For this review, use the dimensioned drawing (mm, ordinates from the lowest corner) and the shaded views. A direction names the side the tool comes from. Coordinates: 2 decimals unless noted, no trailing zeros. Loops run counter-clockwise (first coordinate to the right, second up) from the corner with the lowest first, then second, coordinate; pieces in that order, holes last.
1. Clearance check with a flat-ended pin moving along its axis: P1, Ø1.5, axis at x = 42.5, z = 11.5, coming from the +Y side. State where the tip first meets the part, or that it passes through.
2. Machinability: for the marked faces 4, 5 and 6, which of the approach directions +Z, -Z, +X, -X, +Y, -Y give a long, thin tool a straight path to every point of the face, cutting with its end or side? Answer none if there is none.
3. Take a section at D-D, the plane z = 23.25. State the section outline as (x, y) points, then the cut area to 3 significant figures.
4. Take a section at A-A, the plane x = 7.5. State the section outline as (y, z) points, then the cut area to 3 significant figures.
5. Take a section at B-B, the plane z = 19.5. State the section outline as (x, y) points, then the cut area to 3 significant figures.
6. To check wall thickness, follow probe 1 along Z at (x, y) = (44.5, 5.75); probe 2 along X at (y, z) = (4.25, 17.5); probe 3 along Y at (x, z) = (43.5, 12). State the ranges of each line that lie inside material, in increasing order.
7. Take a section at C-C, the plane y = 0.5. State the section outline as (x, z) points, then the cut area to 3 significant figures.
8. Mouldability with a two-part tool opening along Z and no side actions: class the marked faces 1, 2 and 3 as pulls with the +Z half, pulls with the -Z half, needs draft (parallel to the pull), parting line crosses it, or undercut.
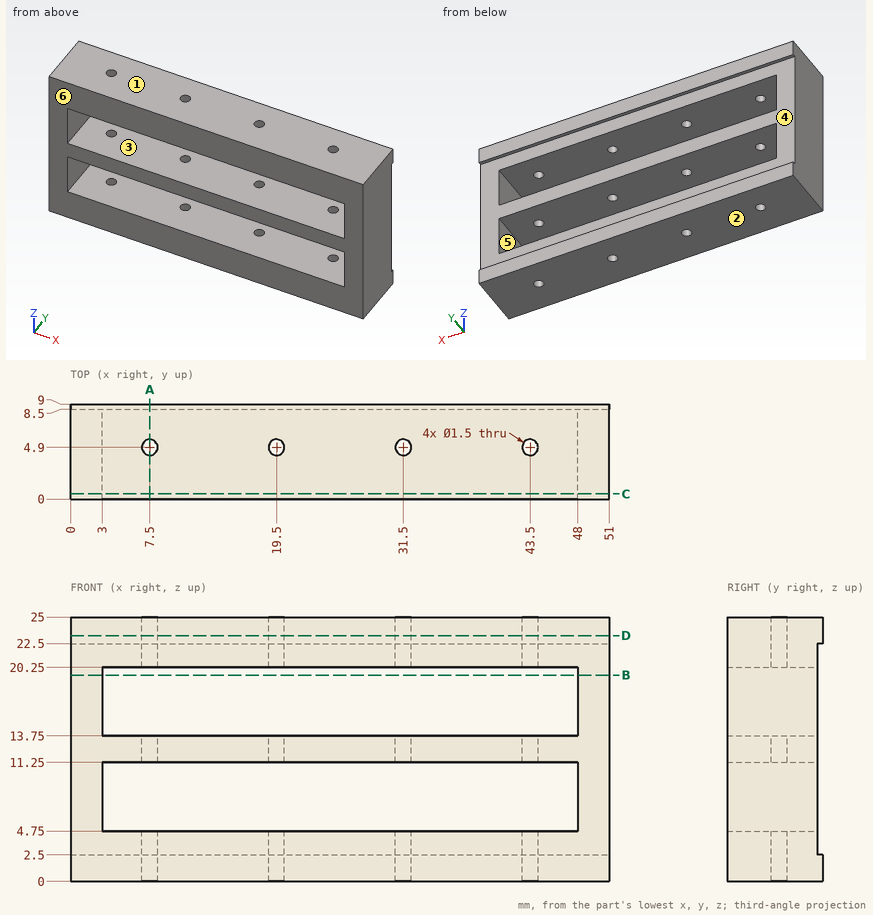
Results list:
1. P1: stops at y = 8.5
2. face 4: +X, -X, +Y
2. face 5: +Y, -Y
2. face 6: +Z, -Z, +X, -X, -Y
3. outline: (0, 0) - (51, 0) - (51, 9) - (0, 9) - close; hole circle Ø1.5 at (7.5, 4.9); hole circle Ø1.5 at (19.5, 4.9); hole circle Ø1.5 at (31.5, 4.9); hole circle Ø1.5 at (43.5, 4.9)
3. area: 452 mm2
4. outline: (0, 0) - (4.15, 0) - (4.15, 4.75) - (0, 4.75) - close; (0, 11.25) - (4.15, 11.25) - (4.15, 13.75) - (0, 13.75) - close; (0, 20.25) - (4.15, 20.25) - (4.15, 25) - (0, 25) - close; (5.65, 0) - (9, 0) - (9, 2.5) - (8.5, 2.5) - (8.5, 4.75) - (5.65, 4.75) - close; (5.65, 11.25) - (8.5, 11.25) - (8.5, 13.75) - (5.65, 13.75) - close; (5.65, 20.25) - (8.5, 20.25) - (8.5, 22.5) - (9, 22.5) - (9, 25) - (5.65, 25) - close
4. area: 86.5 mm2
5. outline: (0, 0) - (3, 0) - (3, 8.5) - (0, 8.5) - close; (48, 0) - (51, 0) - (51, 8.5) - (48, 8.5) - close
5. area: 51.0 mm2
6. probe 1: z = 0 to 4.75, 11.25 to 13.75, 20.25 to 25
6. probe 2: x = 0 to 3, 48 to 51
6. probe 3: y = 0 to 4.15, 5.65 to 8.5
7. outline: (0, 0) - (51, 0) - (51, 25) - (0, 25) - close; hole (3, 4.75) - (48, 4.75) - (48, 11.25) - (3, 11.25) - close; hole (3, 13.75) - (48, 13.75) - (48, 20.25) - (3, 20.25) - close
7. area: 690 mm2
8. face 1: pulls with the +Z half
8. face 2: pulls with the -Z half
8. face 3: undercut
